The model under review builds one solid part; all positions refer to its coordinate system, in mm. Coordinates: 2 decimals unless noted, no trailing zeros. Write each loop counter-clockwise with the first axis right and the second up, starting at its lowest first coordinate (ties: lowest second). Pieces come first, ordered by that corner, then holes. Notation, with made-up numbers: (53, 65) - (75, 65) arc R25 cw to (75, 93) - close; hole circle Ø3 at (40.25, 28.5). An arc over 180 degrees is marked (long way). Put each result on its own line as item: value. Start each with the question number.
Item 1: For pin 1 (12 mm diameter, centred on x = 30, y = 54, fed in from -Z); pin 2 (2 mm diameter, centred on x = 40, y = 3.5, fed in from +Z), all flat-tipped, find the tip position at first contact; note any pin that passes through.
Item 2: Consider section D-D on y = 61.5. Give the boundary of the cut face in (x, z).
Item 3: Consider section A-A on y = 3.5. Give the boundary of the cut face in (x, z).
Item 4: Consider section B-B on x = 15. Give the boundary of the cut face in (y, z), then the cut area to 3 significant figures.
Item 5: Consider section C-C on z = 0.5. Give the boundary of the cut face in (x, y).
Item 6: To check wall thickness, follow L1, parallel to Y at x = 40, z = 2.25; L2, parallel to Y at x = 15, z = 0.7; L3, parallel to X at y = 5, z = 1.85. State the ranges of each line that lie inside material, in increasing order. Write a range as [from, to].
```python
from build123d import *

# Parameters (mm, degrees)
SKETCH1_W           = 92.65
SKETCH1_H           = 65
SKETCH1_R           = 3
SKETCH1_R_2         = 1.35
BOSS_EXTRUDE1_DEPTH = 3
SKETCH2_R           = 1.35
CUT_EXTRUDE1_DEPTH  = 4
SKETCH3_W           = 17
SKETCH3_H           = 15
CUT_EXTRUDE2_DEPTH  = 4
SKETCH4_R           = 3
CUT_EXTRUDE3_DEPTH  = 4


with BuildPart() as part:
    # Sketch1 → Boss-Extrude1 (new body)
    with BuildSketch(Plane.XY):
        with Locations((46.325, 32.5)):
            Rectangle(SKETCH1_W, SKETCH1_H)
        with Locations((15, 53)):
            Circle(SKETCH1_R, mode=Mode.SUBTRACT)
        with Locations((40, 61.5)):
            Circle(SKETCH1_R_2, mode=Mode.SUBTRACT)
        with Locations((40, 3.5)):
            Circle(SKETCH1_R_2, mode=Mode.SUBTRACT)
    extrude(amount=BOSS_EXTRUDE1_DEPTH)

    # Sketch2 → Cut-Extrude1 (cut, through all)
    with BuildSketch(Plane.XY.offset(3)):
        with Locations((89, 61.5)):
            Circle(SKETCH2_R)
        with Locations((89, 3.5)):
            Circle(SKETCH2_R)
    extrude(amount=-CUT_EXTRUDE1_DEPTH, mode=Mode.SUBTRACT)

    # Sketch3 → Cut-Extrude2 (cut, through all)
    with BuildSketch(Plane.XY.offset(3)):
        with Locations((64.15, 7.5)):
            Rectangle(SKETCH3_W, SKETCH3_H)
    extrude(amount=-CUT_EXTRUDE2_DEPTH, mode=Mode.SUBTRACT)

    # Sketch4 → Cut-Extrude3 (cut, through all)
    with BuildSketch(Plane(origin=(0, 0, 0), x_dir=(-1, 0, 0), z_dir=(0, 0, -1))):
        with Locations((-15, 12)):
            Circle(SKETCH4_R)
    extrude(amount=-CUT_EXTRUDE3_DEPTH, mode=Mode.SUBTRACT)


solid = part.part
```
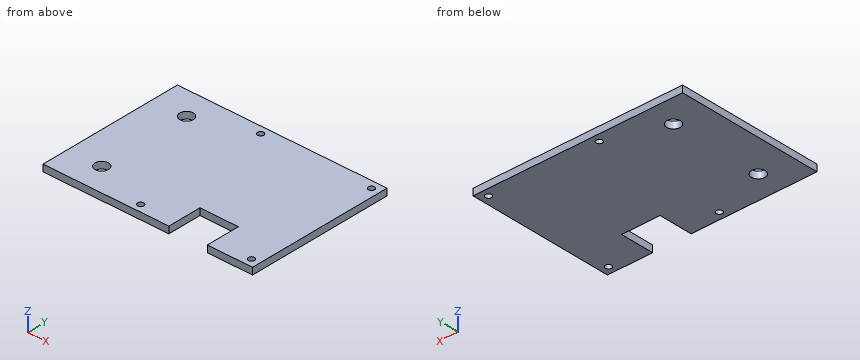
Report:
1. pin 1: z = 0
1. pin 2: through
2. outline: (0, 0) - (38.65, 0) - (38.65, 3) - (0, 3) - close; (41.35, 0) - (87.65, 0) - (87.65, 3) - (41.35, 3) - close; (90.35, 0) - (92.65, 0) - (92.65, 3) - (90.35, 3) - close
3. outline: (0, 0) - (38.65, 0) - (38.65, 3) - (0, 3) - close; (41.35, 0) - (55.65, 0) - (55.65, 3) - (41.35, 3) - close; (72.65, 0) - (87.65, 0) - (87.65, 3) - (72.65, 3) - close; (90.35, 0) - (92.65, 0) - (92.65, 3) - (90.35, 3) - close
4. outline: (0, 0) - (9, 0) - (9, 3) - (0, 3) - close; (15, 0) - (50, 0) - (50, 3) - (15, 3) - close; (56, 0) - (65, 0) - (65, 3) - (56, 3) - close
4. area: 159 mm²
5. outline: (0, 0) - (55.65, 0) - (55.65, 15) - (72.65, 15) - (72.65, 0) - (92.65, 0) - (92.65, 65) - (0, 65) - close; hole circle Ø6 at (15, 12); hole circle Ø6 at (15, 53); hole circle Ø2.7 at (40, 3.5); hole circle Ø2.7 at (40, 61.5); hole circle Ø2.7 at (89, 3.5); hole circle Ø2.7 at (89, 61.5)
6. L1: [0, 2.15], [4.85, 60.15], [62.85, 65]
6. L2: [0, 9], [15, 50], [56, 65]
6. L3: [0, 55.65], [72.65, 92.65]
